```python
from build123d import *

# Parameters (mm, degrees)
F0_R     = 22.5
F0_R_2   = 14.25
F1_DEPTH = 45
F2_SIZE2 = 1.7632698071
F2_SIZE  = 10
F3_R     = 20
F4_R     = 3


with BuildPart() as f1:
    # F0 (on Top) → F1 (new body)
    with BuildSketch(Plane.XY):
        Circle(F0_R)
        Circle(F0_R_2, mode=Mode.SUBTRACT)
    extrude(amount=F1_DEPTH)

    # F2
    f2_edges = [f1.edges().sort_by_distance(p)[0] for p in [
        (-22.5, 0, 0),
        (-22.5, 0, 45),
    ]]
    f2_side = f1.faces().sort_by_distance((-22.5, 0, 22.5))[0]
    chamfer(f2_edges, length=F2_SIZE, length2=F2_SIZE2, reference=f2_side)

    # F3
    f3_edges = [f1.edges().sort_by_distance(p)[0] for p in [
        (22.5, 0, 22.5),
        (-22.5, 0, 10),
        (-22.5, 0, 35),
    ]]
    fillet(f3_edges, radius=F3_R)

    # F4
    f4_edges = [f1.edges().sort_by_distance(p)[0] for p in [
        (-20.73673, 0, 45),
        (-20.73673, 0, 0),
    ]]
    fillet(f4_edges, radius=F4_R)


solid = f1.part
```
Build history of the part. All positions in model axes, mm. Round coordinates to 2 decimals unless told otherwise and drop trailing zeros. Loops run counter-clockwise (first coordinate to the right, second up) from the corner with the lowest first, then second, coordinate; pieces in that order, holes last.
Item 1: Saw through at A-A (z = 25.5). List the corners of the cut face in (x, y).
Item 2: Drill centre lines: line 1 along Y through (x, z) = (0, 22); line 2 along Y through (x, z) = (10.5, 26.5); line 3 along X through (y, z) = (-6, 26.5). Where is each one in solid material? Low to high.
Item 3: Pin check, flat tips, straight feed: P1, Ø10, axis at y = 13.5, z = 28, coming from the +X side; P2, Ø1, axis at x = 7, z = 9.5, coming from the -Y side; P3, Ø8, axis at y = 14, z = 4.5, coming from the -X side. Stop position of each tip, or through.
Item 4: Saw through at B-B (z = 40). List the corners of the cut face in (x, y), then the cut area to 3 significant figures.
Item 5: Two-plate mould, pull along Y, no slides. Class faces 1 (the face through (13.163, -5.458, 22.185)), 2 (the face through (10.382, -19.961, 22.349)), 3 (the face through (8, -12, 45)): released by +Y, released by -Y, zero draft, split by the parting line, or undercut.
Worked answers:
1. outline: circle Ø45 at (0, 0); hole circle Ø28.5 at (0, 0)
2. line 1: y = -22.5 to -14.25, 14.25 to 22.5
2. line 2: y = -19.9 to -9.63, 9.63 to 19.9
2. line 3: x = -21.69 to -12.93, 12.93 to 21.69
3. P1: stops at x = 20.83
3. P2: stops at y = -21.42
3. P3: stops at x = -19.21
4. outline: circle Ø43.24 at (0, 0); hole circle Ø28.5 at (0, 0)
4. area: 830 mm2
5. face 1: undercut
5. face 2: split by the parting line
5. face 3: zero draft
